The figure shows three views and two pictorial views of one solid part (mm, origin at its lowest corner). Answer the questions. A direction names the side the tool comes from. Coordinates: 2 decimals unless noted, no trailing zeros. Loops run counter-clockwise (first coordinate to the right, second up) from the corner with the lowest first, then second, coordinate; pieces in that order, holes last. Notation, with made-up numbers: M -21.5,-9.5 L 10.5,-9.5 A22 ccw 10.5,12.5 Z; hole C 88.25,-21 d10. An arc over 180 degrees is marked long. Answer as a JSON object with one key per item and string values. Group by question number.
1. A cutting plane is placed at A-A on x = 2.5. Give the vertices of the cut face in (y, z), and give its area (3 significant figures).
2. A cutting plane is placed at C-C on y = 71. Give the vertices of the cut face in (x, z).
3. A cutting plane is placed at B-B on z = 2.5. Give the vertices of the cut face in (x, y), and give its area (3 significant figures).
4. For the marked faces 1 and 2, determine the directions among +Z, -Z, +X, -X, +Y, -Y from which every point of the face is accessible in a straight line to the end or side of a thin tool.
5. Given pin 1 (3 mm diameter, centred on y = 11.5, z = 2, fed in from +X); pin 2 (0.9 mm diameter, centred on x = 2.5, y = 45.5, fed in from -Z); pin 3 (2.5 mm diameter, centred on y = 28, z = 2, fed in from -X), each flat-ended and moving along its own axis, determine where each tip first touches the part or whether it passes through.
6. Straight lines are drawn through the part: L1, parallel to X at y = 15.5, z = 1.55; L2, parallel to Y at x = 3.4, z = 4.7. For each, find the intervals that lie inside material, in ascending order.
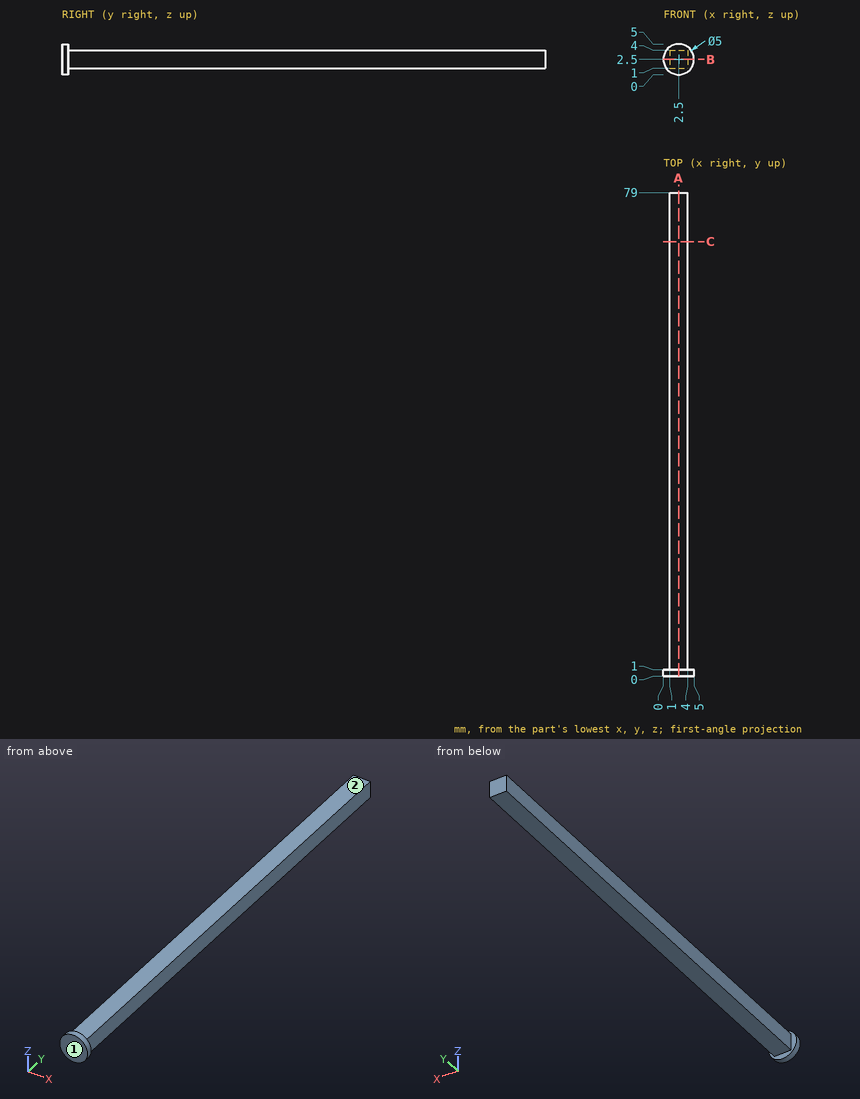
From the geometry:
{
 "1": {"outline": "M 0,0 L 1,0 L 1,1 L 79,1 L 79,4 L 1,4 L 1,5 L 0,5 Z", "area": "239 mm²"},
 "2": {"outline": "M 1,1 L 4,1 L 4,4 L 1,4 Z"},
 "3": {"outline": "M 0,0 L 5,0 L 5,1 L 4,1 L 4,79 L 1,79 L 1,1 L 0,1 Z", "area": "239 mm²"},
 "4": {"face 1": "+Z, -Z, +X, -X, -Y", "face 2": "+Z, +X, -X, +Y"},
 "5": {"pin 1": "stops at x = 4", "pin 2": "stops at z = 1", "pin 3": "stops at x = 1"},
 "6": {"L1": "x = 1 to 4", "L2": "y = 0 to 1"}
}
